from build123d import *

# Parameters (mm, degrees)
SKETCH004_R             = 0.6
SWEEP_ROLL_ANGLE        = -90
CYLINDER006_R           = 0.6
CYLINDER006_DEPTH       = 30
CYLINDER006_PITCH_ANGLE = 90
BOX013_W                = 3.3
BOX013_H                = 7.8
BOX013_DEPTH            = 3.8
BOX012_W                = 30
BOX012_H                = 6.5
BOX012_DEPTH            = 3.8
CUT004_PLACEMENT_ANGLE  = 180


with BuildPart() as sweep_body:
    # Sweep: sweep along a path in Sketch002
    with BuildLine(Plane.XY) as sweep_path:
        Line((0, 0), (2.000007, 0))
        ThreePointArc((2.000007, 0), (3.413537, 0.585387), (3.999404, 1.998718))
        Line((3.999404, 1.998718), (3.999404, 3.99963))
    # Sketch004 → Sweep (sweep)
    with BuildSketch(Plane.YZ):
        Circle(SKETCH004_R)
    sweep(path=sweep_path.line, transition=Transition.RIGHT)


with BuildPart() as sweep_body_1:
    # Sweep roll: moved
    add(sweep_body.part.rotate(Axis((0, 0, 0), (1, 0, 0)), SWEEP_ROLL_ANGLE))


with BuildPart() as sweep_body_2:
    # Sweep placement: moved
    add(sweep_body_1.part.moved(Location((11, 3.4, 2))))


with BuildPart() as fusion002005:
    # Cylinder006 → Cylinder006 (new body)
    with BuildSketch(Plane.XY):
        Circle(CYLINDER006_R)
    extrude(amount=CYLINDER006_DEPTH)


with BuildPart() as fusion002005_1:
    # Cylinder006 pitch: moved
    add(fusion002005.part.rotate(Axis((0, 0, 0), (0, 1, 0)), CYLINDER006_PITCH_ANGLE))


with BuildPart() as fusion002005_2:
    # Cylinder006 placement: moved
    add(fusion002005_1.part.moved(Location((-17, 3.4, 2))))

    # Fusion002005: union Sweep body
    add(sweep_body_2.part)


with BuildPart() as fusion002005_3:
    # Fusion002005 placement: moved
    add(fusion002005_2.part.moved(Location((-1.3, 2.5, 0))))


with BuildPart() as cubo013:
    # Box013 → Box013 (new body)
    with BuildSketch(Plane(origin=(12, -0.5, 0), x_dir=(1, 0, 0), z_dir=(0, 0, 1))):
        with Locations((1.65, 3.9)):
            Rectangle(BOX013_W, BOX013_H)
    extrude(amount=BOX013_DEPTH)


with BuildPart() as cut004:
    # Box012 → Box012 (new body)
    with BuildSketch(Plane(origin=(-18, 0.2, 0), x_dir=(1, 0, 0), z_dir=(0, 0, 1))):
        with Locations((15, 3.25)):
            Rectangle(BOX012_W, BOX012_H)
    extrude(amount=BOX012_DEPTH)

    # Fusion002004: union Cubo013
    add(cubo013.part)

    # Cut004: cut Fusion002005
    add(fusion002005_3.part, mode=Mode.SUBTRACT)


with BuildPart() as cut004_1:
    # Cut004 placement: moved
    add(cut004.part.moved(Location((0.3, -7.1, 1))).rotate(Axis((0.3, -7.1, 1), (0, 0, 1)), CUT004_PLACEMENT_ANGLE))


solid = cut004_1.part
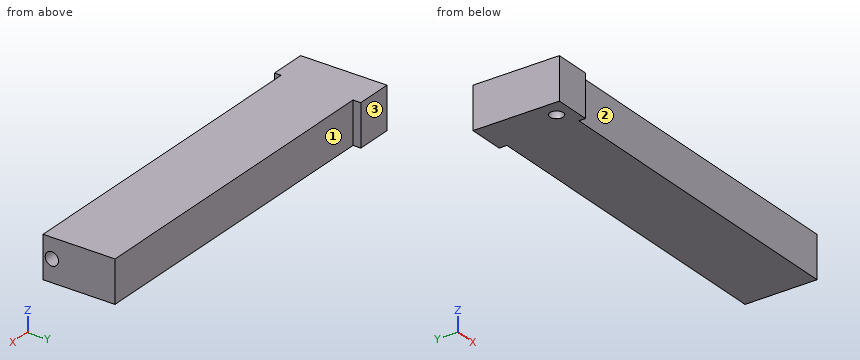
For this review, take the finished solid that the model builds, in its own axes (mm). Face numbers are marked on the shaded views. A direction names the side the tool comes from. Coordinates: 2 decimals unless noted, no trailing zeros. Order: outer loops, then holes, each group sorted by start corner. A loop starts at its lowest first (then second) coordinate and runs counter-clockwise, first axis right, second up. Notation, with made-up numbers: (47.25, 40.25) - (74.25, 40.25) arc R14 cw to (74.25, 44.25) - close; hole circle Ø11 at (33, 83.5). An arc over 180 degrees is marked (long way). Use one line per item in the form item = value.
Q1. Consider section B-B (y = -7). Give the boundary of the cut face in (x, z), then the cut area to 3 significant figures.
Checked values:
outline = (-15, 1) - (-11.7, 1) - (-11.7, 4.8) - (-15, 4.8) - close
area = 12.5 mm2
Q2. For P1, Ø1.1, axis at x = -2.5, z = 3, coming from the +Y side, flat-tipped, find the tip position at first contact; note if it passes through.
Checked values:
P1 = -7.3
Q3. For the marked faces 1, 2 and 3, list the 3-axis set-ups (+Z, -Z, +X, -X, +Y, -Y) from which the entire face can be reached by the end or side of a thin tool; tool diameter is ignored.
Checked values:
face_1 = +Z, -Z, +X, +Y
face_2 = +Z, -Z, +X, -Y
face_3 = +Z, -Z, +X, -X, +Y
Q4. Consider section A-A (x = 2). Give the boundary of the cut face in (y, z).
Checked values:
outline = (-13.8, 1) - (-7.3, 1) - (-7.3, 4.8) - (-13.8, 4.8) - close; hole circle Ø1.2 at (-13, 3)
Q5. For probe 1 along Y at (x, z) = (12, 3); probe 2 along Z at (x, y) = (-0.5, -13); probe 3 along Y at (x, z) = (10, 3.75), list the stretches that pass through material, from the lowest coordinate up. Write a range as from..to.
Checked values:
probe_1 = -13.8..-13.6, -12.4..-7.3
probe_2 = 1..2.4, 3.6..4.8
probe_3 = -13.8..-7.3
